Model file for the job. Use its own axes, mm. A direction names the side the tool comes from. Round coordinates to 2 decimals unless told otherwise and drop trailing zeros. Order: outer loops, then holes, each group sorted by start corner. A loop starts at its lowest first (then second) coordinate and runs counter-clockwise, first axis right, second up. Notation, with made-up numbers: (81.5, -38) -> (139.5, -38) arc R23 cw to (139.5, -15) -> close; hole circle Ø9 at (75.5, 40.5). An arc over 180 degrees is marked (long way). Answer as CSV lines item,"result".
```python
from build123d import *

# Parameters (mm, degrees)
SKETCH_1_W      = 17.13
SKETCH_1_H      = 16.13
EXTRUDE_1_DEPTH = 1
EXTRUDE_2_DEPTH = 2.27
FILLET_1_R      = 0.25


with BuildPart() as part:
    # Эскиз1 → Бобышка-Вытянуть1 (new body)
    with BuildSketch(Plane.XY):
        Rectangle(SKETCH_1_W, SKETCH_1_H)
    extrude(amount=EXTRUDE_1_DEPTH)

    # Эскиз2 → Бобышка-Вытянуть2 (add)
    with BuildSketch(Plane.XY.offset(1)):
        Polygon((4.54, 6.96), (4.54, 2.39), (7.96, 2.39), (7.96, -6.96), (-7.96, -6.96), (-7.96, 6.96), align=None)
    extrude(amount=EXTRUDE_2_DEPTH)

    # Скругление1
    fillet_1_edges = [part.edges().sort_by_distance(p)[0] for p in [
        (-7.96, 0, 3.27),
        (0, -6.96, 3.27),
        (7.96, -2.285, 3.27),
        (6.25, 2.39, 3.27),
        (4.54, 4.675, 3.27),
        (-1.71, 6.96, 3.27),
    ]]
    fillet(fillet_1_edges, radius=FILLET_1_R)


solid = part.part
```
Q1. Saw through at B-B (y = 6.5). Write the cut outline in (x, z) (3 decimals), plus the area to 3 significant figures.
Checks:
outline,"(-8.565, 0) -> (8.565, 0) -> (8.565, 1) -> (4.54, 1) -> (4.54, 3.02) arc R0.25 ccw to (4.29, 3.27) -> (-7.71, 3.27) arc R0.25 ccw to (-7.96, 3.02) -> (-7.96, 1) -> (-8.565, 1) -> close"
area,"45.5 mm²"
Q2. Tool access for faces 1 (the flat face through (0, -6.96, 2)), 2 (the flat face through (7.96, -2, 2)), 3 (the flat face through (4.54, 5, 2)): list every direction of +Z, -Z, +X, -X, +Y, -Y with a clear straight run to the whole face (end or side of a thin tool).
Checks:
face 1,"+Z, +X, -X, -Y"
face 2,"+Z, +X, +Y, -Y"
face 3,"+Z, +X, +Y"
Q3. Saw through at A-A (x = 6). Write the cut outline in (y, z) (3 decimals).
Checks:
outline,"(-8.065, 0) -> (8.065, 0) -> (8.065, 1) -> (2.39, 1) -> (2.39, 3.02) arc R0.25 ccw to (2.14, 3.27) -> (-6.71, 3.27) arc R0.25 ccw to (-6.96, 3.02) -> (-6.96, 1) -> (-8.065, 1) -> close"
Q4. Wall check: L1, parallel to X at y = -2.25, z = 2.5; L2, parallel to Z at x = 5.5, y = -7.25; L3, parallel to Y at x = -5.25, z = 1.8. Give the ranges that are in metal, low to high. Write a range as [from, to].
Checks:
L1,"[-7.96, 7.96]"
L2,"[0, 1]"
L3,"[-6.96, 6.96]"
Q5. Saw through at C-C (z = 1.3). Write the cut outline in (x, y), plus the area to 3 significant figures.
Checks:
outline,"(-7.96, -6.96) -> (7.96, -6.96) -> (7.96, 2.39) -> (4.54, 2.39) -> (4.54, 6.96) -> (-7.96, 6.96) -> close"
area,"206 mm²"
Q6. Flat gauge pins, fed straight in: pin 1 (1 mm diameter, centred on y = -0.5, z = 2.5, fed in from +X); pin 2 (0.6 mm diameter, centred on y = 4, z = 2, fed in from +X); pin 3 (1 mm diameter, centred on y = -3, z = 2.5, fed in from -X); pin 4 (1.6 mm diameter, centred on x = 1.5, z = 1.5, fed in from -Y) (3 decimals). Where does each tip first touch, or does it go through?
Checks:
pin 1,"x = 7.96"
pin 2,"x = 4.54"
pin 3,"x = -7.96"
pin 4,"y = -8.065"
